```python
from build123d import *

# Parameters (mm, degrees)
F0_W     = 146
F0_H     = 46.9
F1_DEPTH = 2
F2_R     = 10
F3_R     = 9.5
F4_DEPTH = 25
F5_R     = 0.1


with BuildPart() as f1:
    # F0 (on Top) → F1 (new body)
    with BuildSketch(Plane.XY):
        Rectangle(F0_W, F0_H)
    extrude(amount=F1_DEPTH)

    # F2
    f2_edges = [f1.edges().sort_by_distance(p)[0] for p in [
        (73, -23.45, 1),
        (73, 23.45, 1),
        (-73, -23.45, 1),
        (-73, 23.45, 1),
    ]]
    fillet(f2_edges, radius=F2_R)

    # F3 (on face) → F4 (cut)
    with BuildSketch(Plane.XY.offset(2)):
        with Locations((0, -1.4277177065)):
            Circle(F3_R)
    extrude(amount=-F4_DEPTH, mode=Mode.SUBTRACT)

    # F5
    f5_edges = [f1.edges().sort_by_distance(p)[0] for p in [
        (73, 0, 2),
        (70.071068, -20.521068, 2),
        (70.071068, 20.521068, 2),
        (0, -23.45, 2),
        (0, 23.45, 2),
        (-70.071068, -20.521068, 2),
        (-70.071068, 20.521068, 2),
        (-73, 0, 2),
        (-9.5, -1.427718, 2),
        (73, 0, 0),
        (70.071068, -20.521068, 0),
        (70.071068, 20.521068, 0),
        (0, -23.45, 0),
        (0, 23.45, 0),
        (-70.071068, -20.521068, 0),
        (-70.071068, 20.521068, 0),
        (-73, 0, 0),
        (-9.5, -1.427718, 0),
    ]]
    fillet(f5_edges, radius=F5_R)


solid = f1.part
```
Could you check a few things on this model? Use its own coordinates, in mm. Coordinates: 2 decimals unless noted, no trailing zeros. Write each loop counter-clockwise with the first axis right and the second up, starting at its lowest first coordinate (ties: lowest second). Pieces come first, ordered by that corner, then holes. Notation, with made-up numbers: M 51,-18 L 102,-18 A26 ccw 102,15 Z; hole C 13,28.5 d2. An arc over 180 degrees is marked long. Answer as CSV lines item,"result". Start each with the question number.
1) I want a section at B-B, the plane z = 1.35. Please give me the cut outline in (x, y), and give its area (3 significant figures).
2) We'd pull the mould along X, two halves only. Please class faces 1 (the cylindrical face through (5.11, 6.58, 1.01)), 2 (the cylindrical face through (-70.15, 20.44, 1.01)), 3 (the flat face through (-1, 11, 2)): +X half, -X half, draft (parallel to the pull), parting line (faces both ways), or undercut.
3) Please list where these lines run through material, in increasing order: line 1 (Y direction, x = 0, z = 1); line 2 (X direction, y = 14, z = 0.45); line 3 (X direction, y = 15, z = 0.35). Write a range as from..to.
4) I want a section at A-A, the plane x = 0. Please give me the cut outline in (y, z), and give its area (3 significant figures).
Data:
1,outline,"M -73,-13.45 A10 ccw -63,-23.45 L 63,-23.45 A10 ccw 73,-13.45 L 73,13.45 A10 ccw 63,23.45 L -63,23.45 A10 ccw -73,13.45 Z; hole C 0,-1.43 d19"
1,area,"6,480 mm^2"
2,face 1,"undercut"
2,face 2,"-X half"
2,face 3,"draft"
3,line 1,"y = -23.45..-10.93, 8.07..23.45"
3,line 2,"x = -72.98..72.98"
3,line 3,"x = -72.88..72.88"
4,outline,"M -23.45,0.1 A0.1 ccw -23.35,0 L -11.03,0 A0.1 ccw -10.93,0.1 L -10.93,1.9 A0.1 ccw -11.03,2 L -23.35,2 A0.1 ccw -23.45,1.9 Z; M 8.07,0.1 A0.1 ccw 8.17,0 L 23.35,0 A0.1 ccw 23.45,0.1 L 23.45,1.9 A0.1 ccw 23.35,2 L 8.17,2 A0.1 ccw 8.07,1.9 Z"
4,area,"55.8 mm^2"
